from build123d import *

# Parameters (mm, degrees)
SKETCH1_W                = 26
SKETCH1_H                = 28
BOSS_EXTRUDE1_DEPTH      = 50
CUT_EXTRUDE3_DEPTH       = 39
SKETCH14_R               = 7.25
BOSS_EXTRUDE7_DEPTH      = 5.8
SKETCH15_R               = 2.8
CUT_EXTRUDE4_DEPTH       = 28
CUT_EXTRUDE7_DEPTH       = 54.29223677
SKETCH19_R               = 2.15
CUT_EXTRUDE9_DEPTH       = 50
ESQUISSE1_W              = 17.371158736
ESQUISSE1_H              = 10.855066753
ENL_V_MAT_EXTRU_1_DEPTH  = 7.5
ENL_V_START              = -7.2
ESQUISSE3_W              = 17.25
ESQUISSE3_H              = 8.423951408
ENL_V_MAT_EXTRU_3_DEPTH  = 7.2
ESQUISSE43_W             = 18.6
ESQUISSE43_H             = 18
ENL_V_MAT_EXTRU_4_DEPTH  = 20
BOSS_EXTRU_28_DEPTH      = 23
ENL_V_MAT_EXTRU_5_DEPTH  = 25
ENL_V_MAT_EXTRU_6_DEPTH  = 7
ESQUISSE48_R             = 4
BOSS_EXTRU_29_DEPTH      = 6
ESQUISSE51_R             = 2.15
ENL_V_MAT_EXTRU_9_DEPTH  = 12
ESQUISSE53_W             = 6.55
ESQUISSE53_H             = 26.2
BOSS_EXTRU_30_DEPTH      = 3.7
ESQUISSE54_W             = 6.55
ESQUISSE54_H             = 26.2
BOSS_EXTRU_31_DEPTH      = 3.7
ESQUISSE55_W             = 3
ESQUISSE55_H             = 25
BOSS_EXTRU_32_DEPTH      = 6.55
ESQUISSE56_R             = 1.15
ESQUISSE56_R_2           = 1.16
ENL_V_MAT_EXTRU_11_DEPTH = 10
CHANFREIN1_SIZE          = 0.7
ESQUISSE57_R             = 2.15
ENL_V_MAT_EXTRU_12_DEPTH = 10
BOSS_EXTRU_33_START      = 1
ESQUISSE58_R             = 1.15
ESQUISSE58_R_2           = 1.16
BOSS_EXTRU_33_DEPTH      = 1
BOSS_EXTRU_34_DEPTH      = 1
ESQUISSE61_W             = 0.45
ESQUISSE61_H             = 6.55
ENL_V_MAT_EXTRU_13_DEPTH = 15
BOSS_EXTRU_35_DEPTH      = 25
ENL_V_MAT_EXTRU_14_DEPTH = 41
ENL_V_MAT_EXTRU_15_DEPTH = 33


with BuildPart() as part:
    # Sketch1 → Boss-Extrude1 (new body)
    with BuildSketch(Plane(origin=(0, 0, 0), x_dir=(1, 0, 0), z_dir=(0, 1, 0))):
        Rectangle(SKETCH1_W, SKETCH1_H)
    extrude(amount=BOSS_EXTRUDE1_DEPTH)

    # Sketch7 → Cut-Extrude3 (cut)
    with BuildSketch(Plane(origin=(13, 0, 0), x_dir=(0, 0, -1), z_dir=(1, 0, 0))):
        with BuildLine():
            Line((4.5, 50), (-14, 50))
            Line((-14, 50), (-14, 24))
            Line((-14, 24), (-0.626524164, 37.373475836))
            ThreePointArc((-0.626524164, 37.373475836), (11.198126611, 39.725545115), (4.5, 49.75))
            Line((4.5, 49.75), (14, 49.75))
            Line((14, 49.75), (14, 50))
            Line((14, 50), (4.5, 50))
        make_face()
    extrude(amount=-CUT_EXTRUDE3_DEPTH, mode=Mode.SUBTRACT)

    # Sketch14 → Boss-Extrude7 (add, symmetric)
    with BuildSketch(Plane(origin=(0, 0, 0), x_dir=(0, 0, -1), z_dir=(1, 0, 0))):
        with Locations((4.5, 42.5)):
            Circle(SKETCH14_R)
    boss_extrude7 = extrude(amount=BOSS_EXTRUDE7_DEPTH, both=True)

    # Symétrie1: Boss-Extrude7 across plane
    add(boss_extrude7.mirror(Plane(origin=(0, 0, 0), x_dir=(0, 0, 1), z_dir=(1, 0, 0))))

    # Sketch15 → Cut-Extrude4 (cut)
    with BuildSketch(Plane(origin=(13, 0, 0), x_dir=(0, 0, -1), z_dir=(1, 0, 0))):
        with Locations((4.5, 42.5)):
            Circle(SKETCH15_R)
    extrude(amount=-CUT_EXTRUDE4_DEPTH, mode=Mode.SUBTRACT)

    # Sketch17 → Cut-Extrude7 (cut, through all)
    with BuildSketch(Plane.XZ):
        Polygon((-9.3, 3.25), (-13, 3.25), (-13, 14), (13, 14), (13, 3.25), (9.3, 3.25), (9.3, 9.8), (-9.3, 9.8), align=None)
    extrude(amount=-CUT_EXTRUDE7_DEPTH, mode=Mode.SUBTRACT)

    # Sketch19 → Cut-Extrude9 (cut)
    with BuildSketch(Plane(origin=(0, 0, -14), x_dir=(-1, 0, 0), z_dir=(0, 0, -1))):
        with Locations((0, 16)):
            Circle(SKETCH19_R)
    extrude(amount=-CUT_EXTRUDE9_DEPTH, mode=Mode.SUBTRACT)

    # Esquisse1 → Enlèv. mat.-Extru.1 (cut)
    with BuildSketch(Plane(origin=(0, 49.75, 0), x_dir=(1, 0, 0), z_dir=(0, 1, 0))):
        with Locations((-14.485579368, 9.927533377)):
            Rectangle(ESQUISSE1_W, ESQUISSE1_H)
    enl_v_mat_extru_1 = extrude(amount=-ENL_V_MAT_EXTRU_1_DEPTH, mode=Mode.SUBTRACT)

    # Symétrie3: Enlèv. mat.-Extru.1 across plane
    add(enl_v_mat_extru_1.mirror(Plane(origin=(0, 0, 0), x_dir=(0, 0, 1), z_dir=(1, 0, 0))), mode=Mode.SUBTRACT)

    # Esquisse3 → Enlèv. mat.-Extru.3 (cut)
    with BuildSketch(Plane(origin=(13, 0, 0), x_dir=(0, 0, -1), z_dir=(1, 0, 0)).offset(ENL_V_START)):
        with Locations((5.375, 38.961975704)):
            Rectangle(ESQUISSE3_W, ESQUISSE3_H)
    enl_v_mat_extru_3 = extrude(amount=ENL_V_MAT_EXTRU_3_DEPTH, mode=Mode.SUBTRACT)

    # Symétrie4: Enlèv. mat.-Extru.3 across plane
    add(enl_v_mat_extru_3.mirror(Plane(origin=(0, 0, 0), x_dir=(0, 0, 1), z_dir=(1, 0, 0))), mode=Mode.SUBTRACT)

    # Esquisse43 → Enlèv. mat.-Extru.4 (cut)
    with BuildSketch(Plane.XY.offset(9.8)):
        with Locations((0, 16)):
            Rectangle(ESQUISSE43_W, ESQUISSE43_H)
    extrude(amount=-ENL_V_MAT_EXTRU_4_DEPTH, mode=Mode.SUBTRACT)

    # Esquisse45 → Boss.-Extru.28 (add)
    with BuildSketch(Plane.XZ):
        Polygon((-9.3, 3.25), (-9.3, 9.8), (9.3, 9.8), (9.3, 3.25), (13, 3.25), (13, -14), (-13, -14), (-13, 3.25), align=None)
    extrude(amount=BOSS_EXTRU_28_DEPTH)

    # Sketch3 → Enlèv. mat.-Extru.5 (cut)
    with BuildSketch(Plane(origin=(0, -23, 0), x_dir=(1, 0, 0), z_dir=(0, 1, 0))):
        Polygon((10, 2.65), (10, 9.85), (2.9, 9.85), (2.9, 5.85), (-2.9, 5.85), (-2.9, 9.85), (-10, 9.85), (-10, 2.65), (-9, 2.65), (-7.502829597, -3.25), (-10, -3.25), (-10, -14.961698536), (10, -14.961698536), (10, -3.25), (7.5, -3.25), (9, 2.65), align=None)
    extrude(amount=ENL_V_MAT_EXTRU_5_DEPTH, mode=Mode.SUBTRACT)

    # Esquisse47 → Enlèv. mat.-Extru.6 (cut)
    with BuildSketch(Plane(origin=(0, 2, 0), x_dir=(-1, 0, 0), z_dir=(0, -1, 0))):
        with BuildLine():
            Line((-9, 2.65), (-9, 5.85))
            Line((-9, 5.85), (-6.550876644, 5.85))
            ThreePointArc((-6.550876644, 5.85), (-2.9, 0.180002706), (-6.550876644, -5.489994589))
            Line((-6.550876644, -5.489994589), (-7.016727392, -5.489994589))
            Line((-7.016727392, -5.489994589), (-9, 2.65))
        make_face()
        with BuildLine():
            Line((6.550876644, 5.85), (9, 5.85))
            Line((9, 5.85), (9, 2.65))
            Line((9, 2.65), (7.016727392, -5.489994589))
            Line((7.016727392, -5.489994589), (6.550876644, -5.489994589))
            ThreePointArc((6.550876644, -5.489994589), (2.9, 0.180002706), (6.550876644, 5.85))
        make_face()
    extrude(amount=-ENL_V_MAT_EXTRU_6_DEPTH, mode=Mode.SUBTRACT)

    # Esquisse48 → Boss.-Extru.29 (add)
    with BuildSketch(Plane.XY.offset(-10.2)):
        with Locations((0, 16)):
            Circle(ESQUISSE48_R)
    extrude(amount=BOSS_EXTRU_29_DEPTH)

    # Esquisse51 → Enlèv. mat.-Extru.9 (cut)
    with BuildSketch(Plane.XY.offset(-5.85)):
        with Locations((0, -8)):
            Circle(ESQUISSE51_R)
    extrude(amount=-ENL_V_MAT_EXTRU_9_DEPTH, mode=Mode.SUBTRACT)

    # Esquisse53 → Boss.-Extru.30 (add)
    with BuildSketch(Plane.ZY.offset(9.3)):
        with Locations((6.525, 15.1)):
            Rectangle(ESQUISSE53_W, ESQUISSE53_H)
    extrude(amount=BOSS_EXTRU_30_DEPTH)

    # Esquisse54 → Boss.-Extru.31 (add)
    with BuildSketch(Plane(origin=(9.3, 0, 0), x_dir=(0, 0, -1), z_dir=(1, 0, 0))):
        with Locations((-6.525, 15.1)):
            Rectangle(ESQUISSE54_W, ESQUISSE54_H)
    extrude(amount=BOSS_EXTRU_31_DEPTH)

    # Esquisse55 → Boss.-Extru.32 (add)
    with BuildSketch(Plane.XY.offset(3.25)):
        with Locations((-11.5, -10.5)):
            Rectangle(ESQUISSE55_W, ESQUISSE55_H)
        with Locations((11.5, -10.5)):
            Rectangle(ESQUISSE55_W, ESQUISSE55_H)
    extrude(amount=BOSS_EXTRU_32_DEPTH)

    # Esquisse56 → Enlèv. mat.-Extru.11 (cut)
    with BuildSketch(Plane.ZY.offset(13)):
        with Locations((-5.2, -14.5)):
            Circle(ESQUISSE56_R)
        with Locations((4.8, -14.5)):
            Circle(ESQUISSE56_R_2)
    extrude(amount=-ENL_V_MAT_EXTRU_11_DEPTH, mode=Mode.SUBTRACT)

    # Chanfrein1
    chanfrein1_edges = [part.edges().sort_by_distance(p)[0] for p in [
        (5.8, 42.5, -1.7),
        (-5.8, 42.5, -1.7),
    ]]
    chamfer(chanfrein1_edges, length=CHANFREIN1_SIZE)

    # Esquisse57 → Enlèv. mat.-Extru.12 (cut)
    with BuildSketch(Plane(origin=(0, 0, -10.2), x_dir=(-1, 0, 0), z_dir=(0, 0, -1))):
        with Locations((0, 16)):
            Circle(ESQUISSE57_R)
    extrude(amount=-ENL_V_MAT_EXTRU_12_DEPTH, mode=Mode.SUBTRACT)

    # Esquisse58 → Boss.-Extru.33 (add)
    with BuildSketch(Plane.ZY.offset(13).offset(BOSS_EXTRU_33_START)):
        Polygon((-14, 34.75), (3.25, 34.75), (3.25, 28.2), (9.8, 28.2), (9.8, -23), (-14, -23), align=None)
        with Locations((-5.2, -14.5)):
            Circle(ESQUISSE58_R, mode=Mode.SUBTRACT)
        with Locations((4.8, -14.5)):
            Circle(ESQUISSE58_R_2, mode=Mode.SUBTRACT)
    extrude(amount=-BOSS_EXTRU_33_DEPTH)

    # Esquisse59 → Boss.-Extru.34 (add)
    with BuildSketch(Plane(origin=(13, 0, 0), x_dir=(0, 0, -1), z_dir=(1, 0, 0))):
        Polygon((-3.25, 28.2), (-3.25, 34.75), (14, 34.75), (14, -23), (-9.8, -23), (-9.8, 28.2), align=None)
    extrude(amount=BOSS_EXTRU_34_DEPTH)

    # Esquisse61 → Enlèv. mat.-Extru.13 (cut)
    with BuildSketch(Plane.XY.offset(3.25)):
        with Locations((-9.075, 31.475)):
            Rectangle(ESQUISSE61_W, ESQUISSE61_H)
        with Locations((9.075, 31.475)):
            Rectangle(ESQUISSE61_W, ESQUISSE61_H)
    extrude(amount=ENL_V_MAT_EXTRU_13_DEPTH, mode=Mode.SUBTRACT)

    # Esquisse62 → Boss.-Extru.35 (add)
    with BuildSketch(Plane.XY.offset(9.8)):
        Polygon((-9.3, 7), (-14, 7), (-14, 28.2), (14, 28.2), (14, 7), (9.3, 7), (9.3, 25), (-9.3, 25), align=None)
    extrude(amount=BOSS_EXTRU_35_DEPTH)

    # Esquisse63 → Enlèv. mat.-Extru.14 (cut)
    with BuildSketch(Plane(origin=(14, 0, 0), x_dir=(0, 0, -1), z_dir=(1, 0, 0))):
        Polygon((-9.8, 7), (-34.636706434, 31.836706434), (-43.129995532, 15.759057015), (-32.785249808, -2.73145904), (-31.803829731, -2.73145904), align=None)
    extrude(amount=-ENL_V_MAT_EXTRU_14_DEPTH, mode=Mode.SUBTRACT)

    # Esquisse64 → Enlèv. mat.-Extru.15 (cut)
    with BuildSketch(Plane.ZY.offset(14)):
        Polygon((31, 28.2), (27.766380883, 28.2), (27.766380883, 24.966380883), align=None)
    extrude(amount=-ENL_V_MAT_EXTRU_15_DEPTH, mode=Mode.SUBTRACT)


solid = part.part
Work out the finished part from the listing and answer in its coordinate system (mm). A direction names the side the tool comes from. Coordinates: 2 decimals unless noted, no trailing zeros. Loops run counter-clockwise (first coordinate to the right, second up) from the corner with the lowest first, then second, coordinate; pieces in that order, holes last. Notation, with made-up numbers: M -28.75,21 L -7.75,21 A18 ccw -7.75,41 Z; hole C 49.25,-18.75 d9. An arc over 180 degrees is marked long. Answer in a Markdown table with one row per item. Add a question column.
1. Consider L1, parallel to X at y = -2.5, z = -9; L2, parallel to Z at x = -9.5, y = -12.5; L3, parallel to Y at x = -12.2, z = 4.8. Determine where each line is inside the solid, lowest interval first.
2. Find section B-B, the plane y = -14.5. Write down the section's boundary in (x, z), then the cut area to 3 significant figures.
3. Find section A-A, the plane x = 0. Write down the section's boundary in (y, z).
4. The mould has two halves that part along Z. Classify faces 1 (the flat face through (-10, -11, -6)), 2 (the flat face through (0, 33, 5)), 3 (the flat face through (10, 34.75, -5)), 4 (the cylindrical face through (0.071, 39.767, -3.893)): pulls with the +Z half, pulls with the -Z half, needs draft (parallel to the pull), parting line crosses it, or undercut.
5. A tool of negligible diameter and unlimited length cuts with its end or side. For faces 5 (the cylindrical face through (-12.028, -14.94, -4.138)), 6 (the flat face through (-9.3, 16, 4)), 7 (the flat face through (-10, -11, 6)), from which of +Z, -Z, +X, -X, +Y, -Y can it reach the whole face along a straight path? Write none if from no direction.
6. Find section D-D, the plane z = 8. Write down the section's boundary in (x, y), then the cut area to 3 significant figures.
7. Flat-ended cylindrical pins translate along their axes: P1, Ø5, axis at x = 0, y = -8, coming from the +Z side; P2, Ø10, axis at x = 5.5, z = 12.5, coming from the -Y side; P3, Ø9, axis at x = -1, y = 16, coming from the +Z side. Find the tip coordinate at first contact, or state that the pin passes through.
8. Find section C-C, the plane x = -11.25. Write down the section's boundary in (y, z).
Reported:
| question | item | result |
|---|---|---|
| 1 | L1 | x = -14 to -10, -2.9 to 2.9, 10 to 14 |
| 1 | L2 | z = -14 to -9.85, -2.65 to 3.25 |
| 1 | L3 | y = -23 to -15.66, -13.34 to 28.2 |
| 2 | outline | M -14,-14 L 14,-14 L 14,9.8 L 10,9.8 L 10,3.25 L 7.5,3.25 L 9,-2.65 L 10,-2.65 L 10,-9.85 L 2.9,-9.85 L 2.9,-5.85 L -2.9,-5.85 L -2.9,-9.85 L -10,-9.85 L -10,-6.35 L -14,-6.35 Z; M -14,-4.05 L -10,-4.05 L -10,-2.65 L -9,-2.65 L -7.5,3.25 L -10,3.25 L -10,3.64 L -14,3.64 Z; M -14,5.96 L -10,5.96 L -10,9.8 L -14,9.8 Z |
| 2 | area | 299 mm^2 |
| 3 | outline | M -23,-14 L -10.15,-14 L -10.15,-5.85 L -23,-5.85 Z; M -5.85,-14 L 13.85,-14 L 13.85,-4.2 L 12,-4.2 L 12,-10.2 L 7,-10.2 L 7,9.8 L 2,9.8 L 2,-5.85 L -5.85,-5.85 Z; M 18.15,-14 L 49.75,-14 L 49.75,-4.5 A7.25 ccw 37.37,0.63 L 28.2,9.8 L 28.2,27.77 L 25,27.77 L 25,-10.2 L 20,-10.2 L 20,-4.2 L 18.15,-4.2 Z; hole C 42.5,-4.5 d5.6 |
| 4 | face 1 | undercut |
| 4 | face 2 | pulls with the +Z half |
| 4 | face 3 | needs draft |
| 4 | face 4 | undercut |
| 5 | face 5 | -X |
| 5 | face 6 | +Z |
| 5 | face 7 | +Z, -Y |
| 6 | outline | M -14,-23 L -10,-23 L -10,2 L 10,2 L 10,-23 L 14,-23 L 14,28.2 L 8.85,28.2 L 8.85,30 L -8.85,30 L -8.85,28.2 L -14,28.2 Z; hole M -9.3,7 L 9.3,7 L 9.3,25 L -9.3,25 Z |
| 6 | area | 631 mm^2 |
| 7 | P1 | stops at z = -5.85 |
| 7 | P2 | stops at y = 2 |
| 7 | P3 | stops at z = -4.2 |
| 8 | outline | M -23,-14 L 34.75,-14 L 34.75,3.25 L 28.2,3.25 L 28.2,27.77 L 24.97,27.77 L 7,9.8 L -23,9.8 Z; hole C -14.5,4.8 d2.32; hole C -14.5,-5.2 d2.3 |
